from build123d import *

# Parameters (mm, degrees)
MODEL_W                 = 3
MODEL_H                 = 3
SALIENTE_EXTRUIR1_DEPTH = 3


with BuildPart() as part:
    # Model → Saliente-Extruir1 (new body)
    with BuildSketch(Plane.XY):
        with BuildLine():
            Line((9.216868636, 295.636684928), (9.216868636, 269.236684928))
            ThreePointArc((9.216868636, 269.236684928), (9.304736602, 269.024552894), (9.516868636, 268.936684928))
            Line((9.516868636, 268.936684928), (12.116868636, 268.936684928))
            Line((12.116868636, 268.936684928), (12.116868636, 266.236684928))
            ThreePointArc((12.116868636, 266.236684928), (12.204736602, 266.024552894), (12.416868637, 265.936684928))
            Line((12.416868637, 265.936684928), (15.016868636, 265.936684928))
            ThreePointArc((15.016868636, 265.936684928), (15.229000671, 266.024552894), (15.316868637, 266.236684928))
            Line((15.316868637, 266.236684928), (15.316868637, 268.936684928))
            Line((15.316868637, 268.936684928), (21.116868637, 268.936684928))
            Line((21.116868637, 268.936684928), (21.116868637, 266.236684928))
            ThreePointArc((21.116868637, 266.236684928), (21.204736602, 266.024552894), (21.416868637, 265.936684928))
            Line((21.416868637, 265.936684928), (24.016868636, 265.936684928))
            ThreePointArc((24.016868636, 265.936684928), (24.229000671, 266.024552894), (24.316868637, 266.236684928))
            Line((24.316868637, 266.236684928), (24.316868637, 268.936684928))
            Line((24.316868637, 268.936684928), (26.916868636, 268.936684928))
            ThreePointArc((26.916868636, 268.936684928), (27.129000671, 269.024552894), (27.216868636, 269.236684928))
            Line((27.216868636, 269.236684928), (27.216868636, 295.636684928))
            ThreePointArc((27.216868636, 295.636684928), (27.129000671, 295.848816963), (26.916868636, 295.936684928))
            Line((26.916868636, 295.936684928), (24.316868637, 295.936684928))
            Line((24.316868637, 295.936684928), (24.316868637, 298.636684928))
            ThreePointArc((24.316868637, 298.636684928), (24.229000671, 298.848816963), (24.016868636, 298.936684928))
            Line((24.016868636, 298.936684928), (21.416868637, 298.936684928))
            ThreePointArc((21.416868637, 298.936684928), (21.204736602, 298.848816963), (21.116868637, 298.636684928))
            Line((21.116868637, 298.636684928), (21.116868637, 295.936684928))
            Line((21.116868637, 295.936684928), (15.316868637, 295.936684928))
            Line((15.316868637, 295.936684928), (15.316868637, 298.636684928))
            ThreePointArc((15.316868637, 298.636684928), (15.229000671, 298.848816963), (15.016868636, 298.936684928))
            Line((15.016868636, 298.936684928), (12.416868637, 298.936684928))
            ThreePointArc((12.416868637, 298.936684928), (12.204736602, 298.848816963), (12.116868636, 298.636684928))
            Line((12.116868636, 298.636684928), (12.116868636, 295.936684928))
            Line((12.116868636, 295.936684928), (9.516868636, 295.936684928))
            ThreePointArc((9.516868636, 295.936684928), (9.304736602, 295.848816963), (9.216868636, 295.636684928))
        make_face()
        with Locations((13.716868636, 291.436684928)):
            Rectangle(MODEL_W, MODEL_H, mode=Mode.SUBTRACT)
        with Locations((22.716868636, 291.436684928)):
            Rectangle(MODEL_W, MODEL_H, mode=Mode.SUBTRACT)
        with Locations((13.716868636, 273.436684928)):
            Rectangle(MODEL_W, MODEL_H, mode=Mode.SUBTRACT)
        with Locations((22.716868636, 273.436684928)):
            Rectangle(MODEL_W, MODEL_H, mode=Mode.SUBTRACT)
        with Locations((13.716868636, 282.436684928)):
            Rectangle(MODEL_W, MODEL_H, mode=Mode.SUBTRACT)
        with Locations((22.716868636, 282.436684928)):
            Rectangle(MODEL_W, MODEL_H, mode=Mode.SUBTRACT)
    extrude(amount=SALIENTE_EXTRUIR1_DEPTH)


solid = part.part
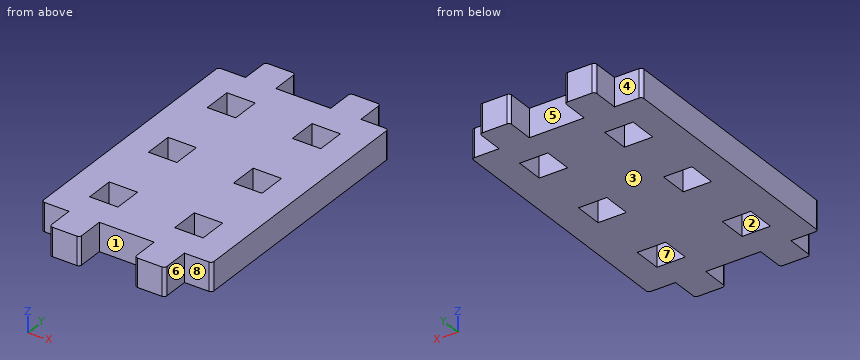
Can you work these out from the model? Positions are in its coordinate system, mm. Face numbers are marked on the shaded views. A direction names the side the tool comes from. Give positions to 0.01 mm unless a question says otherwise; leave off trailing zeros. Loops run counter-clockwise (first coordinate to the right, second up) from the corner with the lowest first, then second, coordinate; pieces in that order, holes last. Notation, with made-up numbers: (-13, -10.75) -> (39, -10.75) arc R19 ccw to (39, 11.25) -> close; hole circle Ø4 at (78.5, 27). An arc over 180 degrees is marked (long way). Write item = value, one per line.
1) Thinking about a two-plate mould opening in X: for the marked faces 5, 6, 7 and 8, which applies, released by +X, released by -X, zero draft, split by the parting line, or undercut?
Check result:
face_5 = undercut
face_6 = released by +X
face_7 = undercut
face_8 = zero draft
2) Suppose I cut it at A-A on x = 22.75. Write out the boundary of the cut face in (y, z), then the cut area to 3 significant figures.
Check result:
outline = (265.94, 0) -> (271.94, 0) -> (271.94, 3) -> (265.94, 3) -> close; (274.94, 0) -> (280.94, 0) -> (280.94, 3) -> (274.94, 3) -> close; (283.94, 0) -> (289.94, 0) -> (289.94, 3) -> (283.94, 3) -> close; (292.94, 0) -> (298.94, 0) -> (298.94, 3) -> (292.94, 3) -> close
area = 72.0 mm2
3) Will these pins go through, and if not, where does the flat tip stop? pin 1 (0.8 mm diameter, centred on x = 25.5, z = 1.5, fed in from -Y); pin 2 (1.5 mm diameter, centred on x = 17.5, z = 2, fed in from +Y).
Check result:
pin_1 = 268.94
pin_2 = 295.94
4) Suppose I cut it at C-C on x = 25. Write out the boundary of the cut face in (y, z).
Check result:
outline = (268.94, 0) -> (295.94, 0) -> (295.94, 3) -> (268.94, 3) -> close
5) For the marked faces 1, 2, 3 and 4, which set-ups out of +Z, -Z, +X, -X, +Y, -Y let a thin tool reach every point of the face, with its end or its side?
Check result:
face_1 = +Z, -Z, -Y
face_2 = +Z, -Z
face_3 = -Z, +X, -X, +Y, -Y
face_4 = +Z, -Z, -X, +Y
6) I need wall thicknesses on L1, parallel to Y at x = 15, z = 1.5; L2, parallel to X at y = 282, z = 0.7; L3, parallel to Y at x = 17.75, z = 2.45. Which ranges of each line are inside material? Lowest first, please. Write a range as from..to.
Check result:
L1 = 265.94..271.94, 274.94..280.94, 283.94..289.94, 292.94..298.94
L2 = 9.22..12.22, 15.22..21.22, 24.22..27.22
L3 = 268.94..295.94
7) Suppose I cut it at B-B on z = 1.15. Give the number of separate pieces and of enclosed holes in the cut face, then the cut area to 3 significant figures.
Check result:
separate_pieces = 1
enclosed_holes = 6
area = 470 mm2
